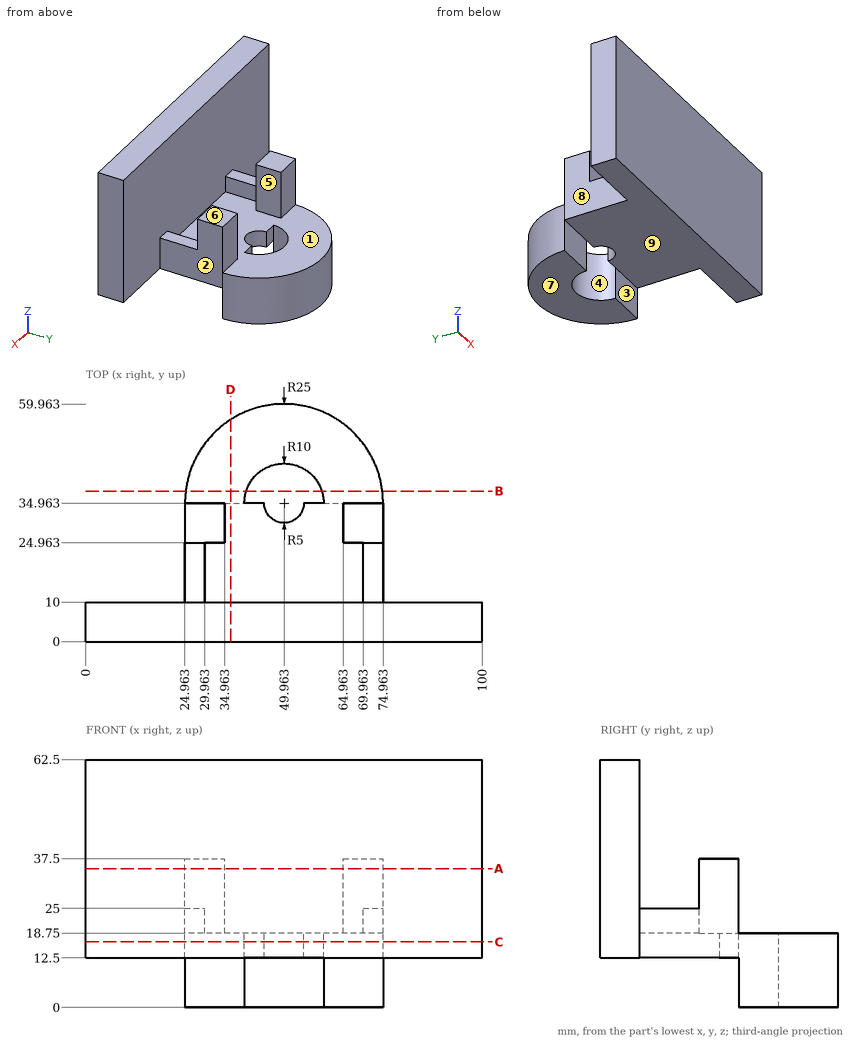
Study the drawing (mm; zero at the part's minimum x, y, z) and answer. A direction names the side the tool comes from. Give positions to 0.01 mm unless a question says otherwise; leave off trailing zeros. Write each loop counter-clockwise with the first axis right and the second up, starting at its lowest first coordinate (ties: lowest second). Pieces come first, ordered by that corner, then holes. Notation, with made-up numbers: (5.25, -20) - (21.25, -20) arc R21 ccw to (21.25, 16) - close; hole circle Ø2 at (79, -16). An arc over 180 degrees is marked (long way). Write item = value, one per line. Start each with the question number.
Item 1: Find section C-C (z = 16.5). Give the vertices of the cut face in (x, y).
Item 2: A tool of negligible diameter and unlimited length cuts with its end or side. For the marked faces 5, 6, 7, 8 and 9, from which of +Z, -Z, +X, -X, +Y, -Y can it reach the whole face along a straight path? Write none if from no direction.
Item 3: Find section D-D (x = 36.5). Give the vertices of the cut face in (y, z).
Item 4: Find section A-A (z = 35). Give the vertices of the cut face in (x, y).
Item 5: Find section B-B (y = 38). Give the vertices of the cut face in (x, z), then the cut area to 3 significant figures.
Item 6: Find the intervals of material crossed by probe 1 along Y at (x, z) = (22, 34.5); probe 2 along X at (y, z) = (11.5, 24.5); probe 3 along X at (y, z) = (24.5, 16), in increasing order. Write a range as [from, to].
Item 7: Each of these flat-tipped pins is pushed along its axis until it touches: P1, Ø4, axis at x = 58.5, z = 15.5, coming from the +Y side; P2, Ø5, axis at x = 65.5, z = 52, coming from the +Y side; P3, Ø7, axis at y = 20.5, z = 22.5, coming from the -X side. Where does it stop, or does it pass through?
Item 8: The mould has two halves that part along X. Classify the marked faces 1, 2, 3 and 4: +X half, -X half, draft (parallel to the pull), parting line (faces both ways), or undercut.
Response:
q1.outline = (0, 0) - (100, 0) - (100, 10) - (74.96, 10) - (74.96, 34.96) arc R25 ccw to (24.96, 34.96) - (24.96, 10) - (0, 10) - close; hole (39.96, 34.96) - (44.96, 34.96) arc R5 ccw to (54.96, 34.96) - (59.96, 34.96) arc R10 ccw to start
q2.face_5 = +Z, +Y
q2.face_6 = +Z, +X, -X, +Y
q2.face_7 = -Z, +X, -X, +Y, -Y
q2.face_8 = +Z, -Z, -X, +Y
q2.face_9 = -Z, +X, -X, -Y
q3.outline = (0, 12.5) - (34.96, 12.5) - (34.96, 0) - (56.03, 0) - (56.03, 18.75) - (10, 18.75) - (10, 62.5) - (0, 62.5) - close
q4.outline = (0, 0) - (100, 0) - (100, 10) - (0, 10) - close; (24.96, 24.96) - (34.96, 24.96) - (34.96, 34.96) - (24.96, 34.96) - close; (64.96, 24.96) - (74.96, 24.96) - (74.96, 34.96) - (64.96, 34.96) - close
q5.outline = (25.15, 0) - (40.44, 0) - (40.44, 18.75) - (25.15, 18.75) - close; (59.49, 0) - (74.78, 0) - (74.78, 18.75) - (59.49, 18.75) - close
q5.area = 573 mm²
q6.probe_1 = [0, 10]
q6.probe_2 = [24.96, 29.96], [69.96, 74.96]
q6.probe_3 = [24.96, 74.96]
q7.P1 = 59.09
q7.P2 = 10
q7.P3 = 24.96
q8.face_1 = undercut
q8.face_2 = +X half
q8.face_3 = draft
q8.face_4 = undercut
